Source: CAD feature listing. Evaluate the final solid. Frame: model axes, mm. Face numbers are marked on the shaded views. Give positions to 0.01 mm unless a question says otherwise; leave off trailing zeros. Order: outer loops, then holes, each group sorted by start corner. A loop starts at its lowest first (then second) coordinate and runs counter-clockwise, first axis right, second up.
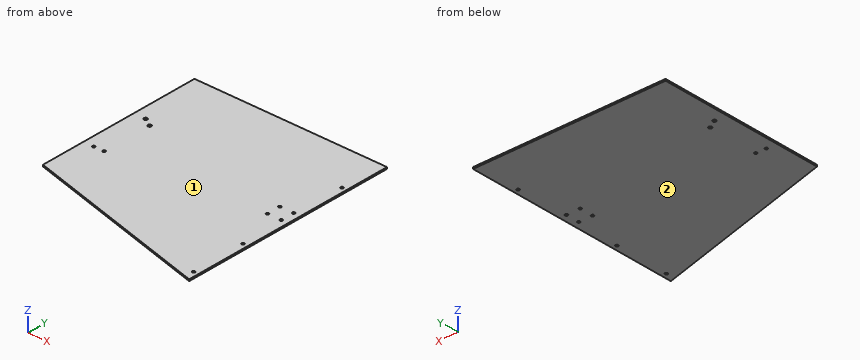
Autodesk Inventor part; units mm, degrees
ref_plane "YZ Plane" through (0, 0, 0) normal (1, 0, 0) x (0, 1, 0)
ref_plane "XZ Plane" through (0, 0, 0) normal (0, 1, 0) x (-1, 0, 0)
ref_plane "XY Plane" through (0, 0, 0) normal (0, 0, 1) x (1, 0, 0)
sketch "Sketch1" plane through (0, 0, 0) normal (0, 0, 1) x (1, 0, 0)
  line L0 (-177.8, 203.2) -> (177.8, 203.2)
  line L1 (177.8, 203.2) -> (177.8, -203.2)
  line L2 (177.8, -203.2) -> (-177.8, -203.2)
  line L3 (-177.8, -203.2) -> (-177.8, 203.2)
  line L4 (-177.8, 203.2) -> (177.8, -203.2) construction
  line L5 (177.8, 203.2) -> (-177.8, -203.2) construction
  point P0 (0, 0)
  dimension "d0" = 355.6
  dimension "d1" = 406.4
extrude "Plate1" add sketch "Sketch1" along normal blind 3.048
sketch "Sketch2" plane through (0, 0, 0) normal (0, 0, -1) x (-1, 0, 0)
  line L0 (177.8, -203.2) -> (-177.8, -203.2) construction
  line L1 (177.8, 203.2) -> (177.8, -203.2) construction
  line L2 (-177.8, 203.2) -> (177.8, 203.2) construction
  line L3 (-177.8, -203.2) -> (-177.8, 203.2) construction
  line L4 (-177.8, -203.2) -> (177.8, -107.9173)
  line L5 (-177.8, -203.2) -> (190.3442, -203.2) construction
  line L6 (177.8, 203.2) -> (177.8, -203.2) construction
  line L7 (177.8, -107.9173) -> (177.8, -203.2)
  line L8 (177.8, -203.2) -> (-177.8, -203.2)
  point P0 (0, 0)
  dimension "d3" = 15
extrude "Cut1" cut sketch "Sketch2" against normal blind 3.048
sketch "Sketch3" plane through (0, 0, 0) normal (0, 0, -1) x (-1, 0, 0)
  line L0 (-177.8, -203.2) -> (177.8, -107.9173) construction
  line L1 (177.8, 203.2) -> (177.8, -107.9173) construction
  line L2 (-177.8, 203.2) -> (177.8, 203.2) construction
  line L3 (-177.8, -203.2) -> (-177.8, 203.2) construction
  line L4 (-177.8, 0) -> (-165.1, 0) construction
  point P0 (0, 0)
  point P1 (-139.7, 0)
  point P2 (-165.1, 25.4)
  point P3 (-139.7, 25.4)
  dimension "d6" = 12.7
  dimension "d9" = 25.4
  dimension "d12" = 25.4
hole "Hole1" at (165.1, 0, 0) at (139.7, 0, 0) at (165.1, 25.4, 0) at (139.7, 25.4, 0) direction (0, 0, 1) diameter 5.1054 end through all
sketch "Sketch4" plane through (0, 0, 0) normal (0, 0, -1) x (-1, 0, 0)
  line L0 (-168.8973, -203.2) -> (-168.8973, 203.2) construction
  line L1 (-177.8, -203.2) -> (-177.8, 203.2)
  point P0 (0, 0)
  point P1 (-168.8973, -184.15)
  point P2 (-168.8973, -82.55)
  point P3 (-168.8973, 120.65)
  dimension "d22" = 8.9027
  dimension "d23" = 101.6
  dimension "d24" = 19.05
  dimension "d25" = 203.2
hole "Hole2" at (168.8973, -184.15, 0) at (168.8973, -82.55, 0) at (168.8973, 120.65, 0) direction (0, 0, 1) diameter 5.1054 end through all
sketch "Sketch5" plane through (0, 0, 0) normal (0, 0, -1) x (-1, 0, 0)
  circle A0 centre (158.75, -25.1401) radius 2.0193
  circle A1 centre (139.7074, -24.6077) radius 2.0193
  point P0 (0, 0)
hole "Hole3" at (-158.75, -25.1401, 0) at (-139.7074, -24.6077, 0) direction (0, 0, 1) diameter 5.1054 depth 3.048 tip angle 118
sketch "Sketch6" plane through (0, 0, 3.048) normal (0, 0, 1) x (1, 0, 0)
  line L0 (-155.0242, 77.8222) -> (-152.7105, 76.4193)
  line L1 (-177.8, -107.9173) -> (-177.8, 203.2)
  point P0 (0, 0)
  point P1 (-155.575, 78.1562)
  point P2 (-139.2858, 68.2788)
  dimension "d40" = 19.05
  dimension "d41" = 22.225
hole "Hole4" at (-155.575, 78.1562, 3.048) at (-139.2858, 68.2788, 3.048) direction (0, 0, -1) diameter 6.35 depth 3.048 tip angle 118
equation "\"d4\" = Thickness"
equation "\"d20\" = Thickness"
equation "\"d31\" = Thickness"
equation "\"d38\" = Thickness"
equation "\"d47\" = Thickness"
equation "\"d2\" = Thickness"
equation "\"BendRadius\" = Thickness"
equation "\"BendReliefWidth\" = Thickness"
equation "\"BendReliefDepth\" = 0.5 * Thickness"
equation "\"CornerReliefSize\" = 4 * Thickness"
equation "\"MinimumRemnant\" = 2 * Thickness"
equation "\"TransitionRadius\" = BendRadius"
equation "\"JacobiRadiusSize\" = BendRadius"
equation "\"GapSize\" = Thickness"
properties part number "hopper_side_l" material "Polycarbonate, Clear"
(1) Line query: line 1 along X through (y, z) = (0, 1.15); line 2 along Y through (x, z) = (165.1, 2.1); line 3 along Y through (x, z) = (-159.5, 2.95). Output: solid intervals per line, ascending.
(2) Draft query along Z for the marked faces 1 and 2. Return one class per face: +Z half, -Z half, draft (parallel to the pull), parting line (faces both ways), or undercut.
(3) Section B-B, the plane x = -22. Return loops of the section in (y, z), plus the area to 3 significant figures.
(4) Pin query (flat end, axial travel): pin 1 Ø1 at (x, y) = (-69, 6) entering from -Z. Return the tip coordinate at first contact, or that it passes through.
(5) Section C-C, the plane x = -110. Return loops of the section in (y, z).
(6) Section A-A, the plane z = 0.85. Count the separate pieces of the cut face and the enclosed holes in it, plus the area to 3 significant figures.
Checks:
1. line 1: x = -177.8 to 137.15, 142.25 to 162.55, 167.65 to 177.8
1. line 2: y = -199.8 to -2.55, 2.55 to 22.85, 27.95 to 203.2
1. line 3: y = -112.82 to -27.58, -22.7 to 203.2
2. face 1: +Z half
2. face 2: -Z half
3. outline: (-149.66, 0) - (203.2, 0) - (203.2, 3.05) - (-149.66, 3.05) - close
3. area: 1,080 mm2
4. pin 1: stops at z = 0
5. outline: (-126.08, 0) - (203.2, 0) - (203.2, 3.05) - (-126.08, 3.05) - close
6. separate pieces: 1
6. enclosed holes: 11
6. area: 127,000 mm2
